Work out the finished part from the listing and answer in its coordinate system (mm). Coordinates: 2 decimals unless noted, no trailing zeros. Order: outer loops, then holes, each group sorted by start corner. A loop starts at its lowest first (then second) coordinate and runs counter-clockwise, first axis right, second up. Notation, with made-up numbers: (-31.5, -19) -> (-2.5, -19) arc R17 cw to (-2.5, 6) -> close; hole circle Ø1 at (58.25, -16.5). An arc over 180 degrees is marked (long way). Write item = value, one per line. Start each with the question number.
Q1. The part is cut by section C-C, the plane z = 6.5. Determine the outline of the cut face in (x, y), plus the area to 3 significant figures.
Q2. For a pull along Y with two mould halves and no side action, classify faces 1 (the cylindrical face through (-14.985, 0.66, 3.954)), 2 (the cylindrical face through (-0.085, 0.644, 1.197)), 3 (the flat face through (3, 0, 0)) as +Y half, -Y half, draft (parallel to the pull), parting line (faces both ways), or undercut.
Q3. Straight lines are drawn through the part: L1, parallel to Y at x = 0, z = 1.25; L2, parallel to Y at x = 0, z = 5.6; L3, parallel to Z at x = 1.75, y = 0. For each, find the intervals that lie inside material, in ascending order. Write a range as from..to.
Q4. Flat-ended cylindrical pins translate along their axes: pin 1 (1 mm diameter, centred on y = 3.5, z = 7, fed in from +X); pin 2 (4 mm diameter, centred on x = -2, y = 4.5, fed in from +Z); pin 3 (3 mm diameter, centred on x = 7.5, z = 7, fed in from -Y); pin 4 (8 mm diameter, centred on x = 8.5, y = -10.5, fed in from -Z). Find the tip coordinate at first contact, or state that the pin passes through.
```python
from build123d import *

# Parameters (mm, degrees)
CYLINDER007_R     = 14
CYLINDER007_DEPTH = 1
CYLINDER006_R     = 14
CYLINDER006_DEPTH = 1
CYLINDER005_R     = 0.4
CYLINDER005_DEPTH = 1
CYLINDER001_R     = 12.6
CYLINDER001_DEPTH = 8
CYLINDER_R        = 15
CYLINDER_DEPTH    = 8
CYLINDER002_R     = 15
CYLINDER002_DEPTH = 1
FILLET_R          = 0.7
FILLET001_R       = 0.7
FILLET002_R       = 0.8
CYLINDER004_R     = 0.4
CYLINDER004_DEPTH = 0.6
CYLINDER003_R     = 0.65
CYLINDER003_DEPTH = 0.6
CHAMFER_SIZE      = 0.2


with BuildPart() as cone001:
    # Cone001 → Cone001 (revolve)
    with BuildSketch(Plane(origin=(0, 0, 7), x_dir=(1, 0, 0), z_dir=(0, -1, 0))):
        Polygon((0, 0), (13.8, 0), (14, 1), (0, 1), align=None)
    revolve(axis=Axis((0, 0, 7), (0, 0, 1)))


with BuildPart() as cone:
    # Cone → Cone (revolve)
    with BuildSketch(Plane(origin=(0, 0, 7), x_dir=(1, 0, 0), z_dir=(0, -1, 0))):
        Polygon((0, 0), (14, 0), (13.8, 1), (0, 1), align=None)
    revolve(axis=Axis((0, 0, 7), (0, 0, 1)))


with BuildPart() as cut005:
    # Cylinder007 → Cylinder007 (new body)
    with BuildSketch(Plane.XY.offset(7)):
        Circle(CYLINDER007_R)
    extrude(amount=CYLINDER007_DEPTH)

    # Cut004: cut Cone
    add(cone.part, mode=Mode.SUBTRACT)

    # Cut005: cut Cone001
    add(cone001.part, mode=Mode.SUBTRACT)


with BuildPart() as cylinder006:
    # Cylinder006 → Cylinder006 (new body)
    with BuildSketch(Plane.XY.offset(7)):
        Circle(CYLINDER006_R)
    extrude(amount=CYLINDER006_DEPTH)


with BuildPart() as cylinder005:
    # Cylinder005 → Cylinder005 (new body)
    with BuildSketch(Plane.XY):
        Circle(CYLINDER005_R)
    extrude(amount=CYLINDER005_DEPTH)


with BuildPart() as cylinder001:
    # Cylinder001 → Cylinder001 (new body)
    with BuildSketch(Plane.XY):
        Circle(CYLINDER001_R)
    extrude(amount=CYLINDER001_DEPTH)


with BuildPart() as cut:
    # Cylinder → Cylinder (new body)
    with BuildSketch(Plane.XY):
        Circle(CYLINDER_R)
    extrude(amount=CYLINDER_DEPTH)

    # Cut: cut Cylinder001
    add(cylinder001.part, mode=Mode.SUBTRACT)


with BuildPart() as fillet002:
    # Cylinder002 → Cylinder002 (new body)
    with BuildSketch(Plane.XY):
        Circle(CYLINDER002_R)
    extrude(amount=CYLINDER002_DEPTH)

    # Fusion: union Cut
    add(cut.part)

    # Cut001: cut Cylinder005
    add(cylinder005.part, mode=Mode.SUBTRACT)

    # Cut003: cut Cylinder006
    add(cylinder006.part, mode=Mode.SUBTRACT)

    # Fillet
    fillet_edges = [fillet002.edges().sort_by_distance(p)[0] for p in [
        (-15, 0, 8),
    ]]
    fillet(fillet_edges, radius=FILLET_R)

    # Fillet001
    fillet001_edges = [fillet002.edges().sort_by_distance(p)[0] for p in [
        (-15, 0, 0),
    ]]
    fillet(fillet001_edges, radius=FILLET001_R)

    # Fillet002
    fillet002_edges = [fillet002.edges().sort_by_distance(p)[0] for p in [
        (-0.4, 0, 0),
    ]]
    fillet(fillet002_edges, radius=FILLET002_R)


with BuildPart() as cylinder004:
    # Cylinder004 → Cylinder004 (new body)
    with BuildSketch(Plane.XY.offset(1)):
        Circle(CYLINDER004_R)
    extrude(amount=CYLINDER004_DEPTH)


with BuildPart() as fusion001:
    # Cylinder003 → Cylinder003 (new body)
    with BuildSketch(Plane.XY.offset(1)):
        Circle(CYLINDER003_R)
    extrude(amount=CYLINDER003_DEPTH)

    # Cut002: cut Cylinder004
    add(cylinder004.part, mode=Mode.SUBTRACT)

    # Chamfer
    chamfer_edges = [fusion001.edges().sort_by_distance(p)[0] for p in [
        (-0.65, 0, 1.6),
    ]]
    chamfer(chamfer_edges, length=CHAMFER_SIZE)

    # Fusion001: union Cut005, Fillet002
    add(cut005.part)
    add(fillet002.part)


solid = fusion001.part
```
Model answer:
q1.outline = circle Ø30 at (0, 0); hole circle Ø25.2 at (0, 0)
q1.area = 208 mm2
q2.face_1 = parting line
q2.face_2 = undercut
q2.face_3 = draft
q3.L1 = -15..-12.6, -0.65..-0.4, 0.4..0.65, 12.6..15
q3.L2 = -15..-12.6, 12.6..15
q3.L3 = 0..1
q4.pin_1 = 14.7
q4.pin_2 = 1
q4.pin_3 = -13.75
q4.pin_4 = 0
